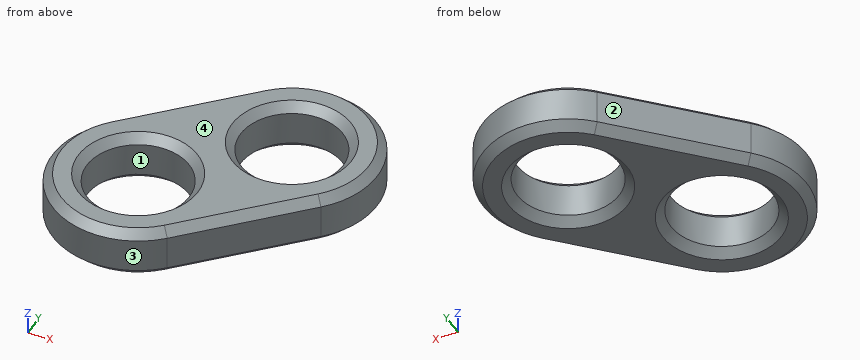
```python
from build123d import *

# Parameters (mm, degrees)
F0_R     = 3
F1_DEPTH = 1.5
F2_SIZE  = 0.5


with BuildPart() as f1:
    # F0 (on Top) → F1 (new body, symmetric)
    with BuildSketch(Plane.XY):
        with BuildLine():
            Line((0.535534, -6.535534), (6.535534, -0.535534))
            ThreePointArc((6.535534, -0.535534), (6.535534, 6.535534), (-0.535534, 6.535534))
            Line((-0.535534, 6.535534), (-6.535534, 0.535534))
            ThreePointArc((-6.535534, 0.535534), (-6.535534, -6.535534), (0.535534, -6.535534))
        make_face()
        with Locations((-3, -3)):
            Circle(F0_R, mode=Mode.SUBTRACT)
        with Locations((3, 3)):
            Circle(F0_R, mode=Mode.SUBTRACT)
    extrude(amount=F1_DEPTH, both=True)

    # F2
    f2_edges = [f1.edges().sort_by_distance(p)[0] for p in [
        (-6, -3, -1.5),
        (-6, -3, 1.5),
        (0, 3, -1.5),
        (3.535534, -3.535534, 1.5),
        (0, 3, 1.5),
        (3.535534, -3.535534, -1.5),
    ]]
    chamfer(f2_edges, length=F2_SIZE)


solid = f1.part
```
Source: CAD feature listing. Evaluate the final solid. Frame: model axes, mm. Face numbers are marked on the shaded views. Coordinates: 2 decimals unless noted, no trailing zeros. Order: outer loops, then holes, each group sorted by start corner. A loop starts at its lowest first (then second) coordinate and runs counter-clockwise, first axis right, second up. Notation, with made-up numbers: (89.25, -29.75) - (110.25, -29.75) arc R18 ccw to (110.25, -7.75) - close; hole circle Ø6 at (19, 71). An arc over 180 degrees is marked (long way). One line per item, written item: value.
1) Cut plane B-B on y = -3. Output: boundary loops of the cut face in (x, z).
Computed values:
outline: (-8, -1) - (-7.5, -1.5) - (-6.5, -1.5) - (-6, -1) - (-6, 1) - (-6.5, 1.5) - (-7.5, 1.5) - (-8, 1) - close; (0, -1) - (0.5, -1.5) - (3.36, -1.5) - (4.07, -1) - (4.07, 1) - (3.36, 1.5) - (0.5, 1.5) - (0, 1) - close
2) Cut plane D-D on z = 1.25. Output: boundary loops of the cut face in (x, y).
Computed values:
outline: (-6.36, 0.36) arc R4.75 ccw to (0.36, -6.36) - (6.36, -0.36) arc R4.75 ccw to (-0.36, 6.36) - close; hole circle Ø6.5 at (-3, -3); hole circle Ø6.5 at (3, 3)
3) Mould query, pull axis X, two halves, no side actions, for the marked faces 1, 2, 3 and 4. Classes: released by +X, released by -X, zero draft, split by the parting line, or undercut.
Computed values:
face 1: undercut
face 2: released by -X
face 3: split by the parting line
face 4: zero draft
4) Contact query for flat-ended pins moving along their axis: pin 1 (3.5 mm diameter, centred on x = -3, y = -3, fed in from +Z); pin 2 (1 mm diameter, centred on y = -4, z = 1, fed in from +X); pin 3 (1 mm diameter, centred on y = 5.5, z = 0, fed in from +X); pin 4 (1.5 mm diameter, centred on x = 5.5, z = 0, fed in from +Y). Output: stop coordinate, or through.
Computed values:
pin 1: passes through
pin 2: stops at x = 3.57
pin 3: stops at x = 7.58
pin 4: stops at y = 7.68
5) Cut plane A-A on z = -0.6. Output: boundary loops of the cut face in (x, y), plus the area to 3 significant figures.
Computed values:
outline: (-6.54, 0.54) arc R5 ccw to (0.54, -6.54) - (6.54, -0.54) arc R5 ccw to (-0.54, 6.54) - close; hole circle Ø6 at (-3, -3); hole circle Ø6 at (3, 3)
area: 107 mm^2
6) Ray query, line 1 (Y direction, x = 3, z = -0.2); line 2 (X direction, y = 0.25, z = 0.5); line 3 (X direction, y = -2, z = -0.85). Return the intervals inside material, ascending. Write a range as [from, to].
Computed values:
line 1: y = [-4.07, 0], [6, 8]
line 2: x = [-6.8, 1.8], [4.2, 7.18]
line 3: x = [-7.9, -5.83], [-0.17, 5.07]
